Autodesk Inventor part; units mm, degrees
ref_plane "Arbeitsebene1" through (30, 0, 0) normal (1, 0, 0) x (0, 1, 0)
ref_plane "XZ Plane" through (0, 0, 0) normal (0, 1, 0) x (-1, 0, 0)
ref_plane "XY Plane" through (0, 0, 0) normal (0, 0, 1) x (1, 0, 0)
sketch "Skizze1" plane through (0, 0, 0) normal (0, 0, 1) x (1, 0, 0)
  line L0 (0, 0) -> (60, 0)
  line L1 (60, 0) -> (60, 60)
  line L2 (60, 60) -> (0, 60)
  line L3 (0, 60) -> (0, 0)
  dimension "d0" = 60
  dimension "d1" = 60
extrude "Extrusion1" add sketch "Skizze1" along normal blind 65
sketch "Skizze2" plane through (0, 0, 65) normal (0, 0, 1) x (1, 0, 0)
  circle A0 centre (30, 30) radius 4
  line L0 (0, 0) -> (60, 0)
  line L1 (0, 60) -> (0, 0)
  dimension "d4" = 8
  dimension "d10" = 30
  dimension "d11" = 30
extrude "Extrusion2" add sketch "Skizze2" along normal blind 10
ref_plane "Arbeitsebene1" through (30, 0, 0) normal (1, 0, 0) x (0, 1, 0)
sketch "Skizze5" plane through (30, 0, 0) normal (1, 0, 0) x (0, 1, 0)
  line L0 (34, 75) -> (26, 75)
  line L1 (30, 75) -> (30, 115)
  line L2 (30, 115) -> (40, 115)
  line L3 (40, 115) -> (40, 112)
  line L4 (38.375, 110.375) -> (40, 112)
  line L5 (38.375, 110.375) -> (38.375, 90.375)
  line L6 (38.375, 90.375) -> (40, 90.375)
  line L7 (40, 90.375) -> (40, 86.375)
  line L8 (40, 86.375) -> (38, 86.375)
  line L9 (38, 86.375) -> (38, 75)
  line L10 (38, 75) -> (30, 75)
  point P0 (0, 0)
  dimension "d25" = 40
  dimension "d26" = 10
  dimension "d27" = 3
  dimension "d30" = 1.625
  dimension "d31" = 135
  dimension "d32" = 20
  dimension "d33" = 4
  dimension "d34" = 2
revolve "Umdrehung1" add sketch "Skizze5" angle 360 about axis through (30, 30, 75) along (0, 0, 1)
sketch "Skizze6" plane through (0, 0, 0) normal (0, 0, -1) x (-1, 0, 0)
  line L0 (0, 0) -> (-60, 0)
  line L1 (0, 0) -> (-7.5, 0)
  line L2 (-7.5, 0) -> (-7.5, 7.5)
  line L3 (-7.5, 7.5) -> (0, 7.5)
  line L4 (0, 7.5) -> (0, 0)
  line L5 (-60, 0) -> (-52.5, 0)
  line L6 (-52.5, 0) -> (-52.5, 7.5)
  line L7 (-52.5, 7.5) -> (-60, 7.5)
  line L8 (-60, 7.5) -> (-60, 0)
  line L9 (-60, 60) -> (0, 60)
  line L10 (-60, 60) -> (-52.5, 60)
  line L11 (-52.5, 60) -> (-52.5, 52.5)
  line L12 (-52.5, 52.5) -> (-60, 52.5)
  line L13 (-60, 52.5) -> (-60, 60)
  line L14 (0, 60) -> (-7.5, 60)
  line L15 (-7.5, 60) -> (-7.5, 52.5)
  line L16 (-7.5, 52.5) -> (0, 52.5)
  line L17 (0, 52.5) -> (0, 60)
  dimension "d36" = 7.5
  dimension "d37" = 7.5
  dimension "d38" = 7.5
  dimension "d39" = 7.5
  dimension "d40" = 7.5
  dimension "d41" = 7.5
  dimension "d42" = 7.5
  dimension "d43" = 7.5
extrude "Extrusion4" cut sketch "Skizze6" against normal blind 60
sketch "Skizze7" plane through (0, 0, 65) normal (0, 0, 1) x (1, 0, 0)
  circle A0 centre (3.75, 3.75) radius 2.25
  circle A1 centre (56.25, 3.75) radius 2.25
  circle A2 centre (56.25, 56.25) radius 2.25
  circle A3 centre (3.75, 56.25) radius 2.25
  point P0 (0, 0)
  dimension "d46" = 4.5
  dimension "d47" = 4.5
  dimension "d48" = 4.5
  dimension "d49" = 4.5
extrude "Extrusion5" cut sketch "Skizze7" against normal blind 5
sketch "Skizze8" plane through (0, 0, 65) normal (0, 0, 1) x (1, 0, 0)
  circle A0 centre (30, 30) radius 8
  circle A1 centre (30, 30) radius 19.075
  point P0 (0, 0)
  dimension "d52" = 38.15
extrude "Extrusion6" add sketch "Skizze8" along normal blind 2.8 contours A0 | A1
properties part number "Motor"
Verification items for the finished model (mm, model axes). A direction names the side the tool comes from. Round coordinates to 2 decimals unless told otherwise and drop trailing zeros. Loops run counter-clockwise (first coordinate to the right, second up) from the corner with the lowest first, then second, coordinate; pieces in that order, holes last. Notation, with made-up numbers: (71, -18.75) - (88, -18.75) arc R13 cw to (88, -10.75) - close; hole circle Ø7 at (-8.75, 19.5). An arc over 180 degrees is marked (long way). Use one line per item in the form item = value.
1. Section check D-D on z = 16.5. Record the cut outline in (x, y), and give its area (4 significant figures).
A:
outline = (0, 7.5) - (7.5, 7.5) - (7.5, 0) - (52.5, 0) - (52.5, 7.5) - (60, 7.5) - (60, 52.5) - (52.5, 52.5) - (52.5, 60) - (7.5, 60) - (7.5, 52.5) - (0, 52.5) - close
area = 3,375 mm²
2. Section check A-A on y = 30. Record the cut outline in (x, z) (3 decimals), and give its area (3 significant figures).
A:
outline = (0, 0) - (60, 0) - (60, 65) - (49.075, 65) - (49.075, 67.8) - (34, 67.8) - (34, 75) - (38, 75) - (38, 86.375) - (40, 86.375) - (40, 90.375) - (38.375, 90.375) - (38.375, 110.375) - (40, 112) - (40, 115) - (20, 115) - (20, 112) - (21.625, 110.375) - (21.625, 90.375) - (20, 90.375) - (20, 86.375) - (22, 86.375) - (22, 75) - (26, 75) - (26, 67.8) - (10.925, 67.8) - (10.925, 65) - (0, 65) - close
area = 4,750 mm²
3. Draft check along Z on faces 1 (the flat face through (5.5, 54.6, 60)), 2 (the flat face through (37, 35, 90.375)), 3 (the cylindrical face through (54, 3.8, 62.5)). Enter one of: pulls with the +Z half, pulls with the -Z half, needs draft (parallel to the pull), parting line crosses it, or undercut.
A:
face_1 = pulls with the -Z half
face_2 = undercut
face_3 = needs draft
4. Section check B-B on x = 3.75. Record the cut outline in (y, z), and give its area (4 significant figures).
A:
outline = (0, 60) - (1.5, 60) - (1.5, 65) - (0, 65) - close; (6, 60) - (7.5, 60) - (7.5, 0) - (52.5, 0) - (52.5, 60) - (54, 60) - (54, 65) - (6, 65) - close; (58.5, 60) - (60, 60) - (60, 65) - (58.5, 65) - close
area = 2,955 mm²
5. Gauge pin test, flat ends, axial feed: pin 1 Ø8 at (x, y) = (6, 20) entering from +Z; pin 2 Ø2 at (x, z) = (3, 44) entering from -Y; pin 3 Ø2 at (x, z) = (5.5, 28) entering from +Y. Record the tip position at first contact, or that the pin passes through.
A:
pin_1 = 65
pin_2 = 7.5
pin_3 = 52.5
6. Access from +Z, -Z, +X, -X, +Y, -Y to the whole of each face (thin tool, end or side, straight path). Record for faces 4 (the cylindrical face through (14.863, 41.607, 66.38)), 5 (the cylindrical face through (29.479, 26.034, 71.35)), 6 (the flat face through (7.5, 4, 30)), 7 (the flat face through (56, 52.5, 30)), 8 (the flat face through (7.5, 56, 30)).
A:
face_4 = +Z
face_5 = none
face_6 = -Z, -X, -Y
face_7 = -Z, +X, +Y
face_8 = -Z, -X, +Y
7. Scan lines: probe 1 along Y at (x, z) = (56, 62); probe 2 along Z at (x, y) = (36, 26.5); probe 3 along X at (y, z) = (3, 63). Record each from-to range of solid material in increasing order.
A:
probe_1 = 0 to 1.51, 5.99 to 54.01, 58.49 to 60
probe_2 = 0 to 67.8, 75 to 115
probe_3 = 0 to 1.63, 5.87 to 54.13, 58.37 to 60
